from build123d import *

# Parameters (mm, degrees)
F0_W     = 250
F0_H     = 88.9
F1_DEPTH = 9.525
F2_R     = 8
F2_R_2   = 2.5
F2_R_3   = 10
F2_R_4   = 3.96875
F3_DEPTH = 25.4


# Not quite as in the source:
# - a pattern or mirror of a feature is missing from the dataset's text; its kind, count and spacing are read off the source's solid


with BuildPart() as f1:
    # F0 (on Front) → F1 (new body, symmetric)
    with BuildSketch(Plane.XZ):
        Rectangle(F0_W, F0_H)
    extrude(amount=F1_DEPTH, both=True)

    # F2 (on face) → F3 (cut)
    with BuildSketch(Plane.XZ.offset(9.525)):
        with Locations((-48, 23.14)):
            Circle(F2_R)
        with Locations((0, 15.95)):
            Circle(F2_R)
        with Locations((-23.5, -7.55)):
            Circle(F2_R_2)
        with Locations((-23.5, 39.45)):
            Circle(F2_R_2)
        with Locations((-97.455, 21.3)):
            Circle(F2_R_3)
        with Locations((-67.85, -25.4)):
            Circle(F2_R_4)
        with Locations((-105.95, -25.4)):
            Circle(F2_R_4)
    f3 = extrude(amount=-F3_DEPTH, mode=Mode.SUBTRACT)

    # F3_copies: F3 across plane
    add(f3.mirror(Plane(origin=(0, 0, 0), x_dir=(0, 0, 1), z_dir=(1, 0, 0))), mode=Mode.SUBTRACT)


solid = f1.part
Here's how the part is built. I have some questions about the finished solid (model axes, mm). Round coordinates to 2 decimals unless told otherwise and drop trailing zeros. Write each loop counter-clockwise with the first axis right and the second up, starting at its lowest first coordinate (ties: lowest second). Pieces come first, ordered by that corner, then holes.
1. I need wall thicknesses on L1, parallel to Z at x = 23.5, y = -5; L2, parallel to Z at x = -48, y = -4.5; L3, parallel to X at y = -6.5, z = 27. Which ranges of each line are inside material? Lowest first, please.
2. Suppose I cut it at B-B (z = -25.4). List the corners of the cut face in (x, y) for me (3 decimals).
3. If we mould it in two halves opening along X, with no side actions, what happens to faces 1 (the cylindrical face through (-105.391, -0.133, 15.215)), 2 (the cylindrical face through (68.71, -0.133, -29.274)), 3 (the flat face through (125, 0, -1)), 4 (the flat face through (-2, 0, 44.45))? For each: released by +X, released by -X, zero draft, split by the parting line, or undercut.
4. Suppose I cut it at D-D (x = -67.85). List the corners of the cut face in (y, z) for me (3 decimals).
5. Suppose I cut it at C-C (y = 6). State how many separate pieces and enclosed holes the cut face has, and give its area (3 significant figures).
6. Suppose I cut it at A-A (x = 23.5). List the corners of the cut face in (y, z) for me (3 decimals), and give its area (3 significant figures).
7. Will this pin go through, and if not, where does the flat tip stop? pin 1 Ø9.5 at (x, z) = (0, 15.95) entering from -Y.
Answer sheet:
1. L1: z = -44.45 to -10.05, -5.05 to 36.95, 41.95 to 44.45
1. L2: z = -44.45 to 15.14, 31.14 to 44.45
1. L3: x = -125 to -105.67, -89.24 to -55.01, -40.99 to 40.99, 55.01 to 89.24, 105.67 to 125
2. outline: (-125, -9.525) - (-109.919, -9.525) - (-109.919, 9.525) - (-125, 9.525) - close; (-101.981, -9.525) - (-71.819, -9.525) - (-71.819, 9.525) - (-101.981, 9.525) - close; (-63.881, -9.525) - (63.881, -9.525) - (63.881, 9.525) - (-63.881, 9.525) - close; (71.819, -9.525) - (101.981, -9.525) - (101.981, 9.525) - (71.819, 9.525) - close; (109.919, -9.525) - (125, -9.525) - (125, 9.525) - (109.919, 9.525) - close
3. face 1: undercut
3. face 2: undercut
3. face 3: released by +X
3. face 4: zero draft
4. outline: (-9.525, -44.45) - (9.525, -44.45) - (9.525, -29.369) - (-9.525, -29.369) - close; (-9.525, -21.431) - (9.525, -21.431) - (9.525, 44.45) - (-9.525, 44.45) - close
5. separate pieces: 1
5. enclosed holes: 13
5. area: 20,700 mm2
6. outline: (-9.525, -44.45) - (9.525, -44.45) - (9.525, -10.05) - (-9.525, -10.05) - close; (-9.525, -5.05) - (9.525, -5.05) - (9.525, 36.95) - (-9.525, 36.95) - close; (-9.525, 41.95) - (9.525, 41.95) - (9.525, 44.45) - (-9.525, 44.45) - close
6. area: 1,500 mm2
7. pin 1: passes through
